Verification items for this drawing (mm, ordinates from the low corner). A direction names the side the tool comes from. Give positions to 0.01 mm unless a question says otherwise; leave off trailing zeros. Loops run counter-clockwise (first coordinate to the right, second up) from the corner with the lowest first, then second, coordinate; pieces in that order, holes last. Notation, with made-up numbers: M 31,-30 L 53,-30 A27 ccw 53,-3 Z; hole C -29.75,22 d6. An arc over 180 degrees is marked long. Use a Markdown table: item, result.
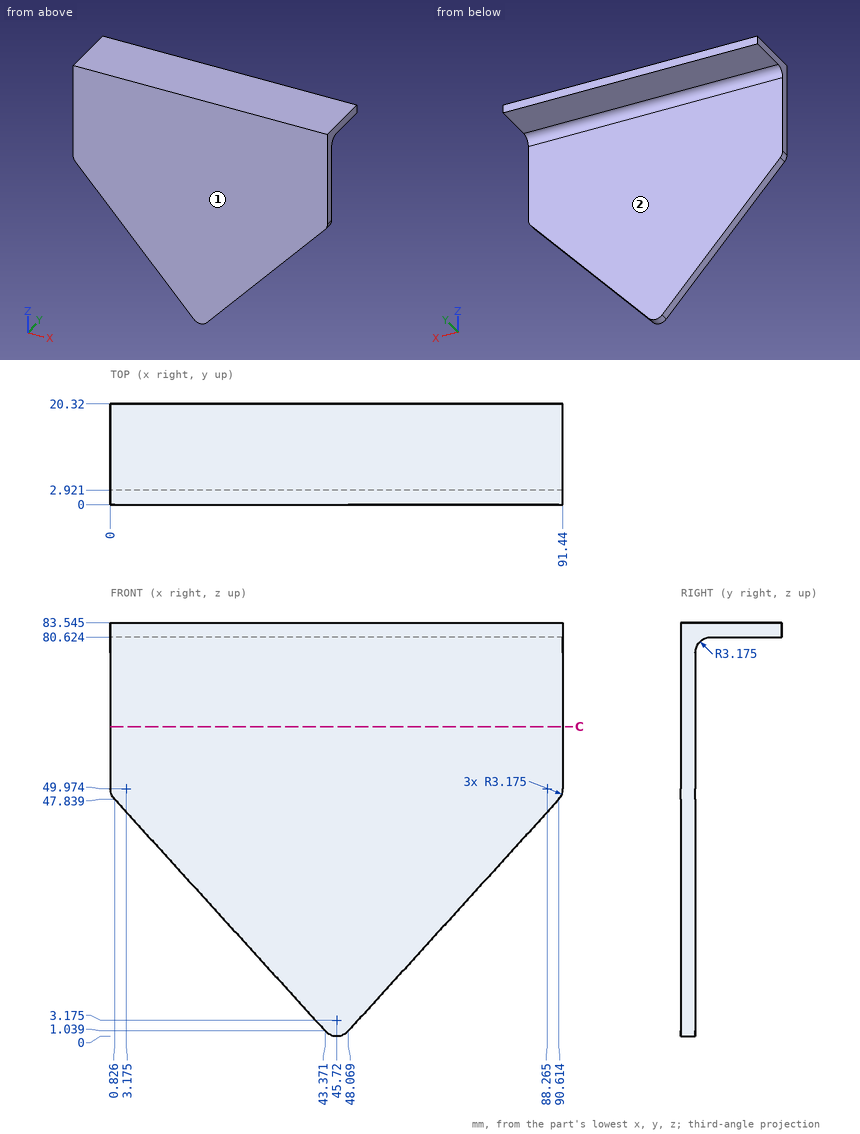
(1) Gauge pin test, flat ends, axial feed: P1, Ø4, axis at x = 12.5, z = 58, coming from the +Y side; P2, Ø4, axis at x = 72.5, y = 3, coming from the -Z side (1 decimal); P3, Ø12, axis at x = 65.5, y = 15.5, coming from the -Z side; P4, Ø3, axis at x = 49, z = 73, coming from the -Y side. Record the tip position at first contact, or that the pin passes through.
Results below:
| item | result |
|---|---|
| P1 | y = 2.92 |
| P2 | z = 25.7 |
| P3 | z = 80.62 |
| P4 | y = 0 |
(2) Set-up check for the marked faces 1 and 2: record each of +Z, -Z, +X, -X, +Y, -Y from which the full face is reachable in a straight line by a thin tool's end or side.
Results below:
| item | result |
|---|---|
| face 1 | +Z, -Z, +X, -X, -Y |
| face 2 | -Z, +X, -X, +Y |
(3) Cross-section at C-C on z = 62.5. Record the cut outline in (x, y).
Results below:
| item | result |
|---|---|
| outline | M 0,0 L 91.44,0 L 91.44,2.92 L 0,2.92 Z |
(4) Material ranges on line 1 (Y direction, x = 58, z = 55.5); line 2 (Z direction, x = 20.5, y = 9) (1 decimal); line 3 (Z direction, x = 30.5, y = 1) (1 decimal), recorded low to high.
Results below:
| item | result |
|---|---|
| line 1 | 0 to 2.92 |
| line 2 | 80.6 to 83.5 |
| line 3 | 15.2 to 83.5 |
